Check sheet for the modelled part. Datum: model origin and axes. Units: mm. A direction names the side the tool comes from. Round coordinates to 2 decimals unless told otherwise and drop trailing zeros. Loops run counter-clockwise (first coordinate to the right, second up) from the corner with the lowest first, then second, coordinate; pieces in that order, holes last. Notation, with made-up numbers: (20, 3.25) - (76, 3.25) arc R25 cw to (76, 37.25) - close; hole circle Ø2 at (48.5, 1.25). An arc over 180 degrees is marked (long way). Put each result on its own line as item: value. Start each with the question number.
Item 1: Section check C-C, the plane x = 75. Record the cut outline in (y, z), and give its area (3 significant figures).
Item 2: Gauge pin test, flat ends, axial feed: pin 1 Ø1 at (y, z) = (41, 5) entering from +X; pin 2 Ø2 at (x, z) = (10.5, 4.5) entering from -Y; pin 3 Ø3 at (y, z) = (-2, 4.5) entering from -X; pin 4 Ø7.5 at (x, y) = (18, 40) entering from +Z. Record the tip position at first contact, or that the pin passes through.
Item 3: Section check B-B, the plane y = 40. Record the cut outline in (x, z) (3 decimals).
Item 4: Section check A-A, the plane x = 18. Record the cut outline in (y, z) (3 decimals).
Item 5: Draft check along Y on faces 5 (the flat face through (63.474, -3, 3)), 6 (the flat face through (42, 0, 3)), 7 (the flat face through (6, 8, 3)). Enter one of: pulls with the +Y half, pulls with the -Y half, needs draft (parallel to the pull), parting line crosses it, or undercut.
Item 6: Section check D-D, the plane y = 29.5. Record the cut outline in (x, z), and give its area (3 significant figures).
Item 7: Tool access check on faces 1 (the flat face through (4, 0, 3)), 2 (the cylindrical face through (1.72, 22.21, 3.13)), 3 (the flat face through (52.527, 10, 3)), 4 (the flat face through (54, 8, 3)). Record the directions out of +Z, -Z, +X, -X, +Y, -Y that give a thin tool (end or side, any length) a straight path to the whole face; none if there is none.
Item 8: Material ranges on line 1 along X through (y, z) = (9, 1.75); line 2 along X through (y, z) = (-1.5, 1.25); line 3 along X through (y, z) = (5, 6.25), recorded low to high.
from build123d import *

# Parameters (mm, degrees)
BOSS_EXTRUDE1_DEPTH = 6.35
SKETCH2_R           = 4.815
CUT_EXTRUDE1_DEPTH  = 6.35
CUT_EXTRUDE2_DEPTH  = 112.983581386
FILLET1_R           = 8


with BuildPart() as part:
    # Sketch1 → Boss-Extrude1 (new body)
    with BuildSketch(Plane.XY):
        Polygon((36.5, 0), (63.4742, 0), (63.4742, -6.35), (75.9742, -6.35), (75.9742, 0), (100, 0), (100, 25), (32, 25), (32, 50), (6, 50), (6, 25), (0, 25), (0, 0), (24, 0), (24, -6.35), (36.5, -6.35), align=None)
    extrude(amount=BOSS_EXTRUDE1_DEPTH)

    # Sketch2 → Cut-Extrude1 (cut)
    with BuildSketch(Plane.XY.offset(6.35)):
        with Locations((18, 40)):
            Circle(SKETCH2_R)
    extrude(amount=-CUT_EXTRUDE1_DEPTH, mode=Mode.SUBTRACT)

    # Sketch3 → Cut-Extrude2 (cut, through all)
    with BuildSketch(Plane.XY.offset(6.35)):
        Polygon((7.9729, 0), (7.9729, 4.7), (5.0138, 4.7), (5.0138, 8), (7.9729, 8), (7.9729, 12.7), (13.0529, 12.7), (13.0529, 8), (16.012, 8), (16.012, 4.7), (13.0529, 4.7), (13.0529, 0), align=None)
        Polygon((47.4471, 12.7), (52.5271, 12.7), (52.5271, 8), (55.4862, 8), (55.4862, 4.7), (52.5271, 4.7), (52.5271, 0), (47.4471, 0), (47.4471, 4.7), (44.488, 4.7), (44.488, 8), (47.4471, 8), align=None)
        Polygon((86.9213, 12.7), (92.0013, 12.7), (92.0013, 8), (94.9604, 8), (94.9604, 4.7), (92.0013, 4.7), (92.0013, 0), (86.9213, 0), (86.9213, 4.7), (83.9622, 4.7), (83.9622, 8), (86.9213, 8), align=None)
    extrude(amount=-CUT_EXTRUDE2_DEPTH, mode=Mode.SUBTRACT)

    # Fillet1
    # the kernel refuses this fillet: 8 mm, written as the material it adds along each edge
    with BuildSketch(Plane(origin=(32, 25, 0), x_dir=(0, 1, 0), z_dir=(0, 0, 1))) as fillet1_piece_1:
        with BuildLine():
            CenterArc((FILLET1_R, -FILLET1_R), FILLET1_R, 90, 90)
            Line((0, -FILLET1_R), (0, 0))
            Line((0, 0), (FILLET1_R, 0))
        make_face()
    extrude(amount=6.35)
    # the kernel refuses this fillet: 8 mm, written as the material it takes off along each edge
    with BuildSketch(Plane(origin=(0, 25, -19.364916731), x_dir=(0, -1, 0), z_dir=(0, 0, 1))) as fillet1_2_piece_1:
        with BuildLine():
            CenterArc((7.745966692, 8), FILLET1_R, 194.477512186, 75.522487814)
            Line((0, 6), (0, 0))
            Line((0, 0), (7.745966692, 0))
        make_face()
    extrude(amount=45.079833462, mode=Mode.SUBTRACT)
    with BuildSketch(Plane(origin=(6, 50, -20), x_dir=(0, -1, 0), z_dir=(0, 0, 1)), Plane(origin=(32, 50, -20), x_dir=(-1, 0, 0), z_dir=(0, 0, 1)), Plane(origin=(100, 25, -20), x_dir=(-1, 0, 0), z_dir=(0, 0, 1))) as fillet1_2_piece_2:
        with BuildLine():
            CenterArc((FILLET1_R, FILLET1_R), FILLET1_R, 180, 90)
            Line((0, FILLET1_R), (0, 0))
            Line((0, 0), (FILLET1_R, 0))
        make_face()
    extrude(amount=46.35, mode=Mode.SUBTRACT)


solid = part.part
Check result:
1. outline: (-6.35, 0) - (25, 0) - (25, 6.35) - (-6.35, 6.35) - close
1. area: 199 mm²
2. pin 1: x = 32
2. pin 2: y = 12.7
2. pin 3: x = 24
2. pin 4: through
3. outline: (6, 0) - (13.185, 0) - (13.185, 6.35) - (6, 6.35) - close; (22.815, 0) - (32, 0) - (32, 6.35) - (22.815, 6.35) - close
4. outline: (0, 0) - (35.185, 0) - (35.185, 6.35) - (0, 6.35) - close; (44.815, 0) - (50, 0) - (50, 6.35) - (44.815, 6.35) - close
5. face 5: needs draft
5. face 6: pulls with the -Y half
5. face 7: undercut
6. outline: (6, 0) - (32.81, 0) - (32.81, 6.35) - (6, 6.35) - close
6. area: 170 mm²
7. face 1: +Z, -Z, -X, -Y
7. face 2: +Z, -Z, -X, +Y
7. face 3: +Z, -Z, -Y
7. face 4: +Z, -Z
8. line 1: 0 to 7.97, 13.05 to 47.45, 52.53 to 86.92, 92 to 100
8. line 2: 24 to 36.5, 63.47 to 75.97
8. line 3: 0 to 5.01, 16.01 to 44.49, 55.49 to 83.96, 94.96 to 100
